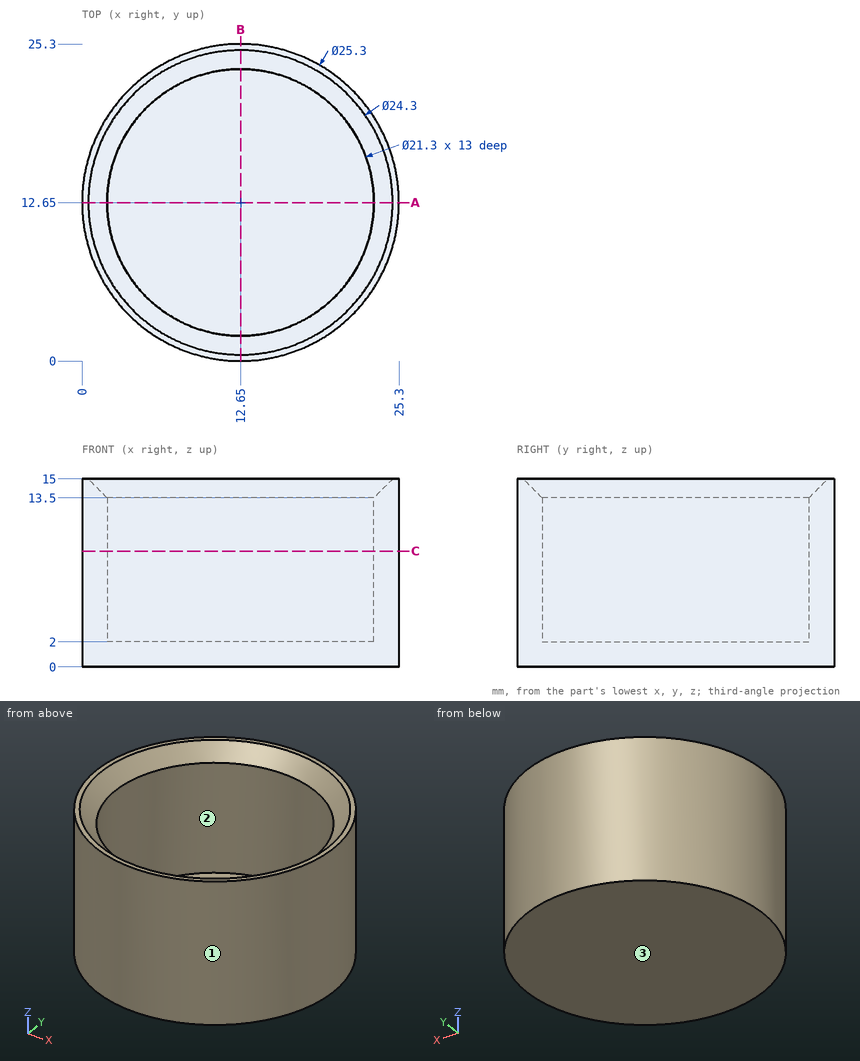
Study the drawing (mm; zero at the part's minimum x, y, z) and answer. Give positions to 0.01 mm unless a question says otherwise; leave off trailing zeros. Loops run counter-clockwise (first coordinate to the right, second up) from the corner with the lowest first, then second, coordinate; pieces in that order, holes last. Notation, with made-up numbers: (-31.5, 63) - (-24.5, 63) arc R21 cw to (-24.5, 94) - close; hole circle Ø4 at (57, 84). An arc over 180 degrees is marked (long way). Answer in a Markdown table with one row per item. Add a question column.
Q1. The part is cut by section A-A (y = 12.65). Determine the outline of the cut face in (x, z), and give its area (3 significant figures).
Q2. Each of these flat-tipped pins is pushed along its axis until it touches: P1, Ø4, axis at y = 8, z = 7, coming from the +X side; P2, Ø4, axis at x = 12, z = 8.5, coming from the +Y side; P3, Ø2, axis at y = 5, z = 4, coming from the +X side; P4, Ø1, axis at y = 20, z = 12.5, coming from the +X side. Where does it stop, or does it pass through?
Q3. The part is cut by section C-C (z = 9.25). Determine the outline of the cut face in (x, y).
Q4. Determine the mould class of the marked faces 1, 2 and 3 for opening direction Y: released by +Y, released by -Y, zero draft, split by the parting line, or undercut.
Q5. Consider line 1 along Y through (x, z) = (12.65, 11); line 2 along Z through (x, y) = (11.5, 7.25); line 3 along Y through (x, z) = (4, 5.5). Determine where each line is inside the solid, lowest interval first.
Solution:
| question | item | result |
|---|---|---|
| 1 | outline | (0, 0) - (25.3, 0) - (25.3, 15) - (24.8, 15) - (23.3, 13.5) - (23.3, 2) - (2, 2) - (2, 13.5) - (0.5, 15) - (0, 15) - close |
| 1 | area | 100 mm² |
| 2 | P1 | stops at x = 25.02 |
| 2 | P2 | stops at y = 25.3 |
| 2 | P3 | stops at x = 23.41 |
| 2 | P4 | stops at x = 23.28 |
| 3 | outline | circle Ø25.3 at (12.65, 12.65); hole circle Ø21.3 at (12.65, 12.65) |
| 4 | face 1 | split by the parting line |
| 4 | face 2 | undercut |
| 4 | face 3 | zero draft |
| 5 | line 1 | y = 0 to 2, 23.3 to 25.3 |
| 5 | line 2 | z = 0 to 2 |
| 5 | line 3 | y = 3.42 to 6.44, 18.86 to 21.88 |
